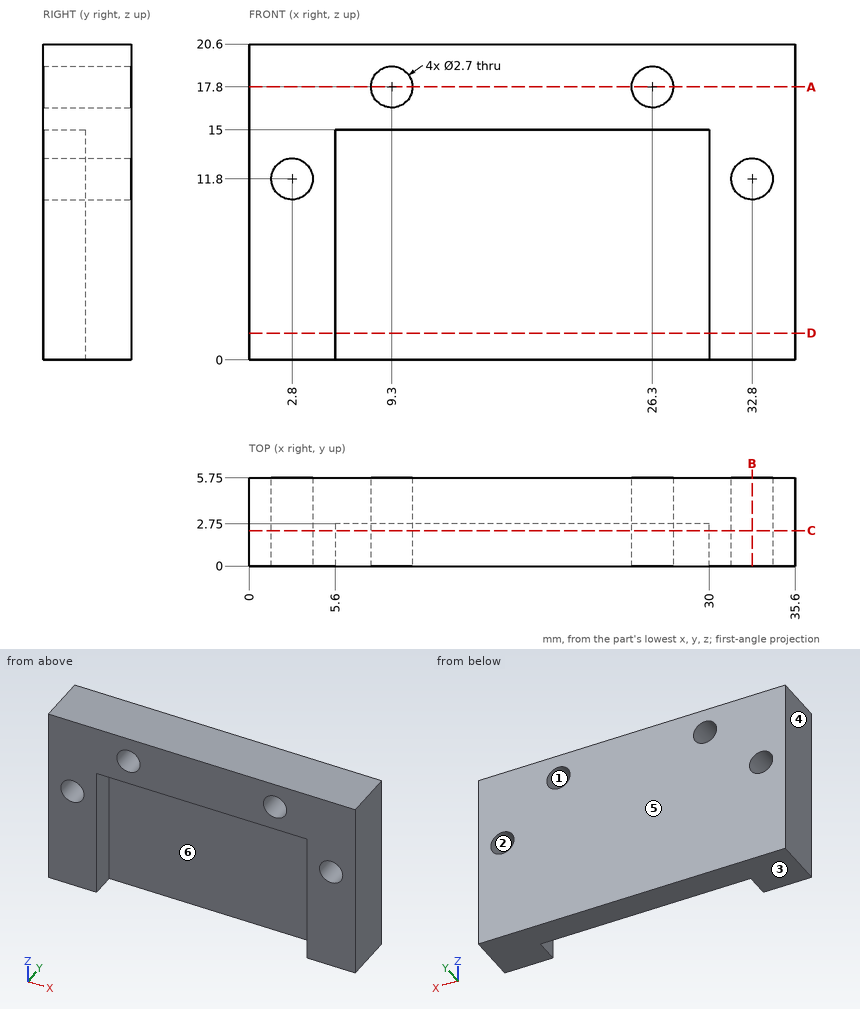
Can you work these out from the drawing? Everything is in mm from the part's minimum corner. A direction names the side the tool comes from. Give positions to 0.01 mm unless a question says otherwise; leave off trailing zeros. Order: outer loops, then holes, each group sorted by start corner. A loop starts at its lowest first (then second) coordinate and runs counter-clockwise, first axis right, second up. Notation, with made-up numbers: M 66.25,69 L 116.25,69 A34 cw 116.25,99 Z; hole C 15,8 d1. An arc over 180 degrees is marked long. Use a Markdown table: item, result. Add a question column.
Item 1: For the marked faces 5 and 6, which set-ups out of +Z, -Z, +X, -X, +Y, -Y let a thin tool reach every point of the face, with its end or its side?
Item 2: Suppose I cut it at A-A (z = 17.8). List the corners of the cut face in (x, y) for me, then the cut area to 3 significant figures.
Item 3: We'd pull the mould along X, two halves only. Please class the marked faces 1, 2, 3 and 4: +X half, -X half, draft (parallel to the pull), parting line (faces both ways), or undercut.
Item 4: Suppose I cut it at B-B (x = 32.8). List the corners of the cut face in (y, z) for me.
Item 5: If I drill on L1, parallel to X at y = 0.85, z = 11.75; L2, parallel to X at y = 3.7, z = 11.8; L3, parallel to X at y = 1.15, z = 6.5, over which ranges is the centre line in solid material (lowest first)? Write a range as [from, to].
Item 6: Suppose I cut it at D-D (z = 1.75). List the corners of the cut face in (x, y) for me, then the cut area to 3 significant figures.
Item 7: Will these pins go through, and if not, where does the flat tip stop? pin 1 (0.8 mm diameter, centred on x = 18.5, y = 1, fed in from -Z); pin 2 (4.5 mm diameter, centred on x = 15.5, z = 4.5, fed in from -Y).
Item 8: Suppose I cut it at C-C (y = 2.3). List the corners of the cut face in (x, z) for me, then the cut area to 3 significant figures.
Answer sheet:
| question | item | result |
|---|---|---|
| 1 | face 5 | +Z, -Z, +X, -X, +Y |
| 1 | face 6 | -Z, -Y |
| 2 | outline | M 0,0 L 7.95,0 L 7.95,5.75 L 0,5.75 Z; M 10.65,0 L 24.95,0 L 24.95,5.75 L 10.65,5.75 Z; M 27.65,0 L 35.6,0 L 35.6,5.75 L 27.65,5.75 Z |
| 2 | area | 174 mm² |
| 3 | face 1 | undercut |
| 3 | face 2 | undercut |
| 3 | face 3 | draft |
| 3 | face 4 | -X half |
| 4 | outline | M 0,0 L 5.75,0 L 5.75,10.45 L 0,10.45 Z; M 0,13.15 L 5.75,13.15 L 5.75,20.6 L 0,20.6 Z |
| 5 | L1 | x = [0, 1.45], [4.15, 5.6], [30, 31.45], [34.15, 35.6] |
| 5 | L2 | x = [0, 1.45], [4.15, 31.45], [34.15, 35.6] |
| 5 | L3 | x = [0, 5.6], [30, 35.6] |
| 6 | outline | M 0,0 L 5.6,0 L 5.6,2.75 L 30,2.75 L 30,0 L 35.6,0 L 35.6,5.75 L 0,5.75 Z |
| 6 | area | 138 mm² |
| 7 | pin 1 | stops at z = 15 |
| 7 | pin 2 | stops at y = 2.75 |
| 8 | outline | M 0,0 L 5.6,0 L 5.6,15 L 30,15 L 30,0 L 35.6,0 L 35.6,20.6 L 0,20.6 Z; hole C 2.8,11.8 d2.7; hole C 9.3,17.8 d2.7; hole C 26.3,17.8 d2.7; hole C 32.8,11.8 d2.7 |
| 8 | area | 344 mm² |
